Study the drawing (mm; zero at the part's minimum x, y, z) and answer. A direction names the side the tool comes from. Coordinates: 2 decimals unless noted, no trailing zeros. Loops run counter-clockwise (first coordinate to the right, second up) from the corner with the lowest first, then second, coordinate; pieces in that order, holes last. Notation, with made-up numbers: (44.25, 87.25) -> (68.25, 87.25) arc R25 ccw to (68.25, 102.25) -> close; hole circle Ø5 at (-16, 61.25). An arc over 180 degrees is marked (long way). Answer as a JSON object with one key per item and string values. Group by question number.
Q1. The part is cut by section D-D on z = 15.75. Write down the section's boundary in (x, y), and give its area (3 significant figures).
Q2. The part is cut by section B-B on y = 86. Write down the section's boundary in (x, z), and give its area (3 significant figures).
Q3. For the marked faces 1 and 2, determine the directions among +Z, -Z, +X, -X, +Y, -Y from which every point of the face is accessible in a straight line to the end or side of a thin tool.
Q4. The part is cut by section C-C on y = 63.5. Write down the section's boundary in (x, z), and give its area (3 significant figures).
Q5. The part is cut by section A-A on x = 63.5. Write down the section's boundary in (y, z).
Q6. Each of these flat-tipped pins is pushed along its axis until it touches: P1, Ø5, axis at x = 92.5, y = 16, coming from the +Z side; P2, Ø4, axis at x = 54.5, z = 8, coming from the +Y side; P3, Ø2, axis at y = 42.5, z = 4, coming from the +X side. Where does it stop, or does it pass through?
Q7. Straight lines are drawn through the part: line 1 along Y through (x, z) = (63.5, 3.4); line 2 along Z through (x, y) = (83, 101); line 3 along X through (y, z) = (63, 16.5). For each, find the intervals that lie inside material, in ascending order. Write a range as [from, to].
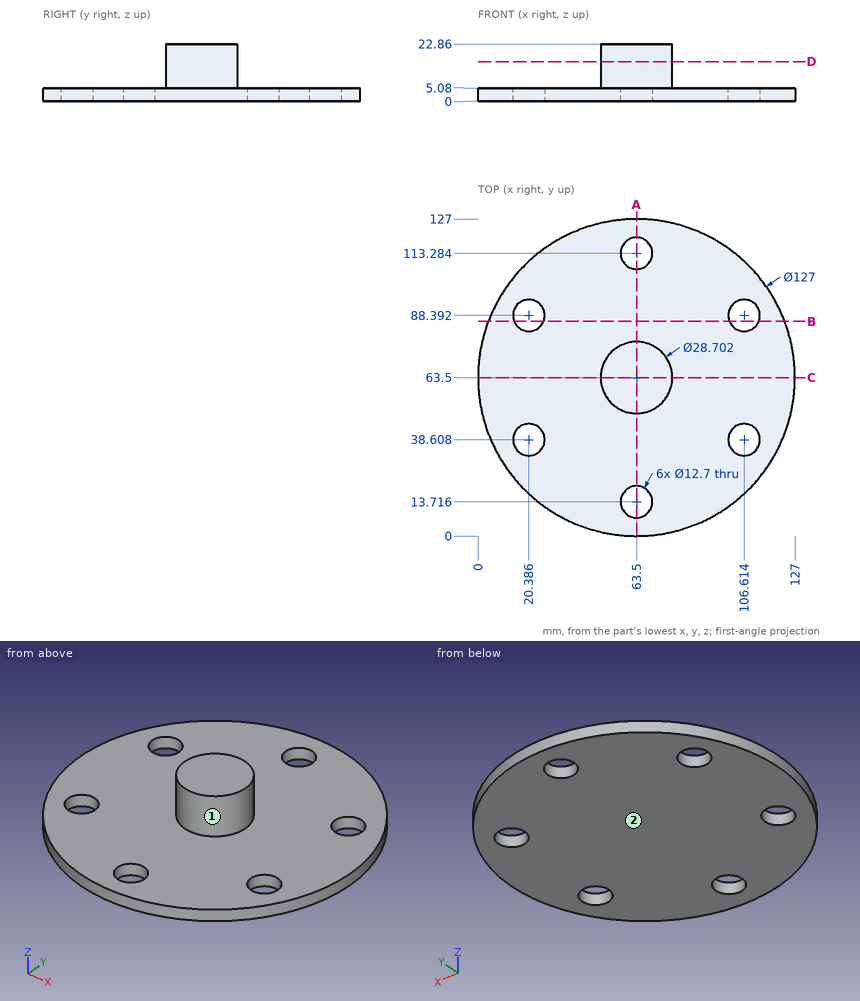
Final values:
{
 "1": {"outline": "circle Ø28.7 at (63.5, 63.5)", "area": "647 mm2"},
 "2": {"outline": "(4.12, 0) -> (14.5, 0) -> (14.5, 5.08) -> (4.12, 5.08) -> close; (26.27, 0) -> (100.73, 0) -> (100.73, 5.08) -> (26.27, 5.08) -> close; (112.5, 0) -> (122.88, 0) -> (122.88, 5.08) -> (112.5, 5.08) -> close", "area": "484 mm2"},
 "3": {"face 1": "+Z", "face 2": "-Z, +X, -X, +Y, -Y"},
 "4": {"outline": "(0, 0) -> (127, 0) -> (127, 5.08) -> (77.85, 5.08) -> (77.85, 22.86) -> (49.15, 22.86) -> (49.15, 5.08) -> (0, 5.08) -> close", "area": "1,160 mm2"},
 "5": {"outline": "(0, 0) -> (7.37, 0) -> (7.37, 5.08) -> (0, 5.08) -> close; (20.07, 0) -> (106.93, 0) -> (106.93, 5.08) -> (77.85, 5.08) -> (77.85, 22.86) -> (49.15, 22.86) -> (49.15, 5.08) -> (20.07, 5.08) -> close; (119.63, 0) -> (127, 0) -> (127, 5.08) -> (119.63, 5.08) -> close"},
 "6": {"P1": "stops at z = 5.08", "P2": "stops at y = 76.03", "P3": "stops at x = 123.77"},
 "7": {"line 1": "y = [0, 7.37], [20.07, 106.93], [119.63, 127]", "line 2": "z = [0, 5.08]", "line 3": "x = [49.16, 77.84]"}
}
